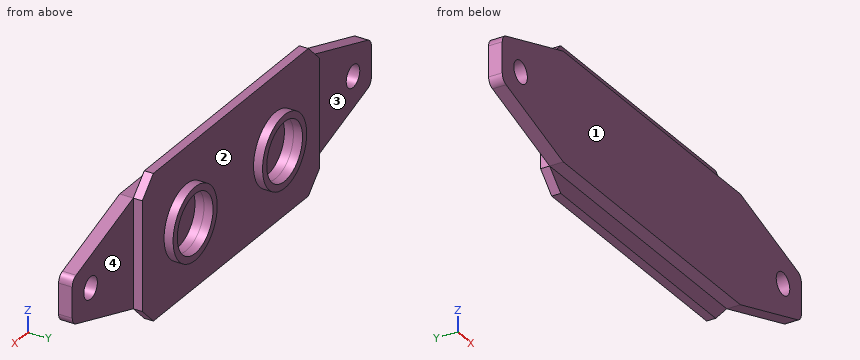
```python
from build123d import *

# Parameters (mm, degrees)
EXTRUDE1_DEPTH = 3.175
SKETCH5_R      = 12.6587948
SKETCH5_R_2    = 10.263887676
EXTRUDE2_DEPTH = 3.175
SKETCH7_R      = 10.263887676
EXTRUDE3_DEPTH = 114.636616568
SKETCH8_R      = 3.888872997
SKETCH8_W      = 50.8
SKETCH8_H      = 38.1
EXTRUDE4_DEPTH = 4.7752


with BuildPart() as part:
    # Sketch4 → Extrude1 (new body)
    with BuildSketch(Plane(origin=(0, 0, 0), x_dir=(1, 0, 0), z_dir=(0, 1, 0))):
        Polygon((0, 44.45), (6.35, 50.8), (95.25, 50.8), (101.6, 44.45), (101.6, 6.35), (95.25, 0), (6.35, 0), (0, 6.35), align=None)
    extrude(amount=-EXTRUDE1_DEPTH)

    # Sketch5 → Extrude2 (add)
    # profile 1 of 2: a face of its own
    with BuildSketch(Plane(origin=(0, 0, 0), x_dir=(1, 0, 0), z_dir=(0, 1, 0))):
        with Locations(Location((25.140280811, 25.4, 0), (0, 0, 90))):
            Circle(SKETCH5_R)
        with Locations(Location((25.140280811, 25.4, 0), (0, 0, 270))):
            Circle(SKETCH5_R_2, mode=Mode.SUBTRACT)
    # profile 2 of 2: a face of its own
    with BuildSketch(Plane(origin=(0, 0, 0), x_dir=(1, 0, 0), z_dir=(0, 1, 0))):
        with Locations(Location((76.459719189, 25.4, 0), (0, 0, 90))):
            Circle(SKETCH5_R)
        with Locations(Location((76.459719189, 25.4, 0), (0, 0, 90))):
            Circle(SKETCH5_R_2, mode=Mode.SUBTRACT)
    extrude(amount=EXTRUDE2_DEPTH)

    # Sketch7 → Extrude3 (cut, through all)
    with BuildSketch(Plane(origin=(0, 0, 0), x_dir=(1, 0, 0), z_dir=(0, 1, 0))):
        with Locations(Location((25.140280811, 25.4, 0), (0, 0, 270))):
            Circle(SKETCH7_R)
        with Locations(Location((76.459719189, 25.4, 0), (0, 0, 90))):
            Circle(SKETCH7_R)
    extrude(amount=-EXTRUDE3_DEPTH, mode=Mode.SUBTRACT)

    # Sketch8 → Extrude4 (add)
    # profile 1 of 4: a face of its own
    with BuildSketch(Plane(origin=(0, -3.175, 0), x_dir=(-1, 0, 0), z_dir=(0, 1, 0))):
        with BuildLine():
            ThreePointArc((-134.414065233, -33.76600747), (-136.000297004, -32.612437385), (-136.606100968, -30.746999975))
            Line((-136.606100968, -30.746999975), (-136.606100968, -20.053000025))
            ThreePointArc((-136.606100968, -20.053000025), (-136.000297004, -18.187562615), (-134.414065233, -17.03399253))
            Line((-134.414065233, -17.03399253), (-101.6, -6.35))
            Line((-101.6, -6.35), (-101.6, -44.45))
            Line((-101.6, -44.45), (-134.414065233, -33.76600747))
        make_face()
        with Locations(Location((-126.068509621, -25.4, 0), (0, 0, 90))):
            Circle(SKETCH8_R, mode=Mode.SUBTRACT)
    # profile 2 of 4: a face of its own
    with BuildSketch(Plane(origin=(0, -3.175, 0), x_dir=(-1, 0, 0), z_dir=(0, 1, 0))):
        with Locations((-76.2, -25.4)):
            Rectangle(SKETCH8_W, SKETCH8_H)
    # profile 3 of 4: a face of its own
    with BuildSketch(Plane(origin=(0, -3.175, 0), x_dir=(-1, 0, 0), z_dir=(0, 1, 0))):
        with Locations((-25.4, -25.4)):
            Rectangle(SKETCH8_W, SKETCH8_H)
    # profile 4 of 4: a face of its own
    with BuildSketch(Plane(origin=(0, -3.175, 0), x_dir=(-1, 0, 0), z_dir=(0, 1, 0))):
        with BuildLine():
            ThreePointArc((32.814065233, -17.03399253), (34.400297004, -18.187562615), (35.006100968, -20.053000025))
            Line((35.006100968, -20.053000025), (35.006100968, -30.746999975))
            ThreePointArc((35.006100968, -30.746999975), (34.400297004, -32.612437385), (32.814065233, -33.76600747))
            Line((32.814065233, -33.76600747), (0, -44.45))
            Line((0, -44.45), (0, -6.35))
            Line((0, -6.35), (32.814065233, -17.03399253))
        make_face()
        with Locations(Location((24.468509621, -25.4, 0), (0, 0, 90))):
            Circle(SKETCH8_R, mode=Mode.SUBTRACT)
    extrude(amount=-EXTRUDE4_DEPTH)


solid = part.part
```
The listing builds one solid part. Answer for the finished solid, in the listing's coordinates (mm). Face numbers are marked on the shaded views. A direction names the side the tool comes from. Give positions to 0.01 mm unless a question says otherwise; leave off trailing zeros. Loops run counter-clockwise (first coordinate to the right, second up) from the corner with the lowest first, then second, coordinate; pieces in that order, holes last. Notation, with made-up numbers: M 44,72.25 L 74,72.25 A28 ccw 74,109.25 Z; hole C 33,54.25 d9. An arc over 180 degrees is marked long. One line per item, written item: value.
Q1. For the marked faces 3 and 4, determine the directions among +Z, -Z, +X, -X, +Y, -Y from which every point of the face is accessible in a straight line to the end or side of a thin tool.
Working result:
face 3: +Z, -Z, -X, +Y
face 4: +Z, -Z, +X, +Y
Q2. Determine the mould class of the marked faces 1 and 2 for opening direction X: +X half, -X half, draft (parallel to the pull), parting line (faces both ways), or undercut.
Working result:
face 1: draft
face 2: undercut
Q3. A cutting plane is placed at B-B on x = 9. Determine the outline of the cut face in (y, z) (3 decimals).
Working result:
outline: M -7.95,-44.45 L -3.175,-44.45 L -3.175,-50.8 L 0,-50.8 L 0,0 L -3.175,0 L -3.175,-6.35 L -7.95,-6.35 Z
Q4. A cutting plane is placed at A-A on z = -25.4. Give the number of separate pieces and of enclosed holes in the cut face, then the cut area to 3 significant figures.
Working result:
separate pieces: 3
enclosed holes: 0
area: 968 mm^2
Q5. A cutting plane is placed at C-C on z = -42.5. Determine the outline of the cut face in (x, y) (3 decimals), then the cut area to 3 significant figures.
Working result:
outline: M -5.989,-7.95 L 107.589,-7.95 L 107.589,-3.175 L 101.6,-3.175 L 101.6,0 L 0,0 L 0,-3.175 L -5.989,-3.175 Z
area: 865 mm^2
Q6. Find the intervals of material crossed by line 1 (X direction, y = -6.25, z = -25.4); line 2 (X direction, y = -0.95, z = -25.4); line 3 (Z direction, x = 32, y = -5.5), in increasing order. Write a range as from..to.
Working result:
line 1: x = -35.01..-28.36, -20.58..122.18, 129.96..136.61
line 2: x = 0..14.88, 35.4..66.2, 86.72..101.6
line 3: z = -44.45..-6.35
Q7. Flat-ended cylindrical pins translate along their axes: P1, Ø5.5, axis at x = 33.5, y = -5.5, coming from the +Z side; P2, Ø1.9, axis at x = 64.5, z = -4, coming from the -Y side (3 decimals); P3, Ø1.5, axis at x = -4.5, y = -1, coming from the +Z side; P4, Ø3, axis at x = 103.5, y = -2.5, coming from the -Z side. Find the tip coordinate at first contact, or state that the pin passes through.
Working result:
P1: stops at z = 0
P2: stops at y = -3.175
P3: passes through
P4: stops at z = -44.27
Q8. A cutting plane is placed at D-D on x = 73. Determine the outline of the cut face in (y, z) (3 decimals).
Working result:
outline: M -7.95,-44.45 L -3.175,-44.45 L -3.175,-50.8 L 0,-50.8 L 0,-37.577 L 3.175,-37.577 L 3.175,-35.063 L -3.175,-35.063 L -3.175,-15.737 L 3.175,-15.737 L 3.175,-13.223 L 0,-13.223 L 0,0 L -3.175,0 L -3.175,-6.35 L -7.95,-6.35 Z
